Autodesk Inventor part; units mm, degrees
ref_plane "YZ Plane" through (0, 0, 0) normal (1, 0, 0) x (0, 1, 0)
ref_plane "XZ Plane" through (0, 0, 0) normal (0, 1, 0) x (-1, 0, 0)
ref_plane "XY Plane" through (0, 0, 0) normal (0, 0, 1) x (1, 0, 0)
sketch "Náčrt1" plane through (0, 0, 0) normal (0, 0, 1) x (1, 0, 0)
  line L0 (0, 7) -> (0, -7)
  line L1 (-7, 0) -> (7, 0)
  line L2 (-3.5, 3.5) -> (3.5, 3.5)
  line L3 (3.5, 3.5) -> (3.5, -3.5)
  line L4 (3.5, -3.5) -> (-3.5, -3.5)
  line L5 (-3.5, -3.5) -> (-3.5, 3.5)
  line L6 (-5, 5) -> (5, 5)
  line L7 (5, 5) -> (5, -5)
  line L8 (5, -5) -> (-5, -5)
  line L9 (-5, -5) -> (-5, 5)
  point P0 (0, 0)
  dimension "d1" = 10
  dimension "d2" = 10
  dimension "d3" = 1.5
  dimension "d4" = 1.5
  dimension "d5" = 1.5
  dimension "d6" = 1.5
extrude "Vysunutí1" add sketch "Náčrt1" along normal mid plane 40 contours L6 L7 L1 L3 L2 L0 | L0 L2 L5 L1 L9 L6 | L1 L5 L4 L0 L8 L9 | L7 L8 L0 L4 L3 L1
sketch "Náčrt2" plane through (-5, 5, 20) normal (0, 1, 0) x (1, 0, 0)
  line L0 (12, 20) -> (-2, 20)
  line L1 (5, 48) -> (5, -8)
  line L2 (10, 0) -> (0, 0)
  line L3 (0, 40) -> (0, 0)
  point P0 (5, 20)
  point P1 (5, 5)
  dimension "d10" = 5
  dimension "d11" = 5
hole "Díra1" at (0, 5, 15) direction (0, -1, 0) diameter 3.2 end through all counterbore diameter 6.5 counterbore depth 2
sketch "Náčrt3" plane through (-5, 5, 20) normal (0, 1, 0) x (1, 0, 0)
  line L0 (0, 40) -> (0, 0)
  line L1 (0, 40) -> (10, 40)
  point P0 (5, 20)
  point P1 (5, 34)
  point P2 (5, 22)
  dimension "d19" = 5
  dimension "d20" = 5
  dimension "d21" = 12
  dimension "d22" = 6
hole "Díra2" at (0, 5, -14) at (0, 5, -2) direction (0, -1, 0) diameter 2.459 depth 1.5
properties part number "y_standoff" material "Hliník 6061"
For this review, take the finished solid that the model builds, in its own axes (mm). A direction names the side the tool comes from. Round coordinates to 2 decimals unless told otherwise and drop trailing zeros. Write each loop counter-clockwise with the first axis right and the second up, starting at its lowest first coordinate (ties: lowest second). Pieces come first, ordered by that corner, then holes. Notation, with made-up numbers: (-36, 65.25) -> (0, 65.25) arc R14 ccw to (0, 74.25) -> close; hole circle Ø2 at (78.5, 63.5). An arc over 180 degrees is marked (long way). Use CSV: the item, a comma, the result in double quotes.
(1) Consider section C-C, the plane z = 15. Give the boundary of the cut face in (x, y).
Computed values:
outline,"(-5, -5) -> (-1.6, -5) -> (-1.6, -3.5) -> (-3.5, -3.5) -> (-3.5, 3.5) -> (-3.25, 3.5) -> (-3.25, 5) -> (-5, 5) -> close; (1.6, -5) -> (5, -5) -> (5, 5) -> (3.25, 5) -> (3.25, 3.5) -> (3.5, 3.5) -> (3.5, -3.5) -> (1.6, -3.5) -> close"
(2) Consider section B-B, the plane x = 0. Give the boundary of the cut face in (y, z).
Computed values:
outline,"(-5, -20) -> (-3.5, -20) -> (-3.5, 13.4) -> (-5, 13.4) -> close; (-5, 16.6) -> (-3.5, 16.6) -> (-3.5, 20) -> (-5, 20) -> close; (3.5, -20) -> (5, -20) -> (5, -15.23) -> (3.5, -15.23) -> close; (3.5, -12.77) -> (5, -12.77) -> (5, -3.23) -> (3.5, -3.23) -> close; (3.5, -0.77) -> (5, -0.77) -> (5, 11.75) -> (3.5, 11.75) -> close; (3.5, 18.25) -> (5, 18.25) -> (5, 20) -> (3.5, 20) -> close"
(3) Consider section A-A, the plane y = 3. Give the boundary of the cut face in (x, z).
Computed values:
outline,"(-5, -20) -> (-3.5, -20) -> (-3.5, 20) -> (-5, 20) -> close; (3.5, -20) -> (5, -20) -> (5, 20) -> (3.5, 20) -> close"
(4) Draft analysis for pull direction X (two halves, no side actions). For faces 4 (the face through (-5, 0, 0)), 5 (the face through (-4.5, 0.1, 20)), 6 (the face through (0, 3.5, 0)), state which applies: +X half, -X half, draft (parallel to the pull), parting line (faces both ways), or undercut.
Computed values:
face 4,"-X half"
face 5,"draft"
face 6,"undercut"
(5) To check wall thickness, follow L1, parallel to Z at x = 0, y = 3.85; L2, parallel to X at y = 4.7, z = 15; L3, parallel to X at y = 0.5, z = -5.5. State the ranges of each line that lie inside material, in increasing order. Write a range as [from, to].
Computed values:
L1,"[-20, -15.23], [-12.77, -3.23], [-0.77, 11.75], [18.25, 20]"
L2,"[-5, -3.25], [3.25, 5]"
L3,"[-5, -3.5], [3.5, 5]"
(6) For faces 1 (the face through (0, 5, 0)), 2 (the face through (0, -3.5, 0)), 3 (the face through (-0.369, 4.24, -0.827)), list the 3-axis set-ups (+Z, -Z, +X, -X, +Y, -Y) from which the entire face can be reached by the end or side of a thin tool; tool diameter is ignored.
Computed values:
face 1,"+Z, -Z, +X, -X, +Y"
face 2,"+Z, -Z"
face 3,"+Y"
(7) Clearance check with a flat-ended pin moving along its axis: P1, Ø2, axis at x = 0, z = -2, coming from the +Y side. State where the tip first meets the part, or that it passes through.
Computed values:
P1,"y = -3.5"
(8) Consider section D-D, the plane z = -14. Give the boundary of the cut face in (x, y).
Computed values:
outline,"(-5, -5) -> (5, -5) -> (5, 5) -> (1.23, 5) -> (1.23, 3.5) -> (3.5, 3.5) -> (3.5, -3.5) -> (-3.5, -3.5) -> (-3.5, 3.5) -> (-1.23, 3.5) -> (-1.23, 5) -> (-5, 5) -> close"
